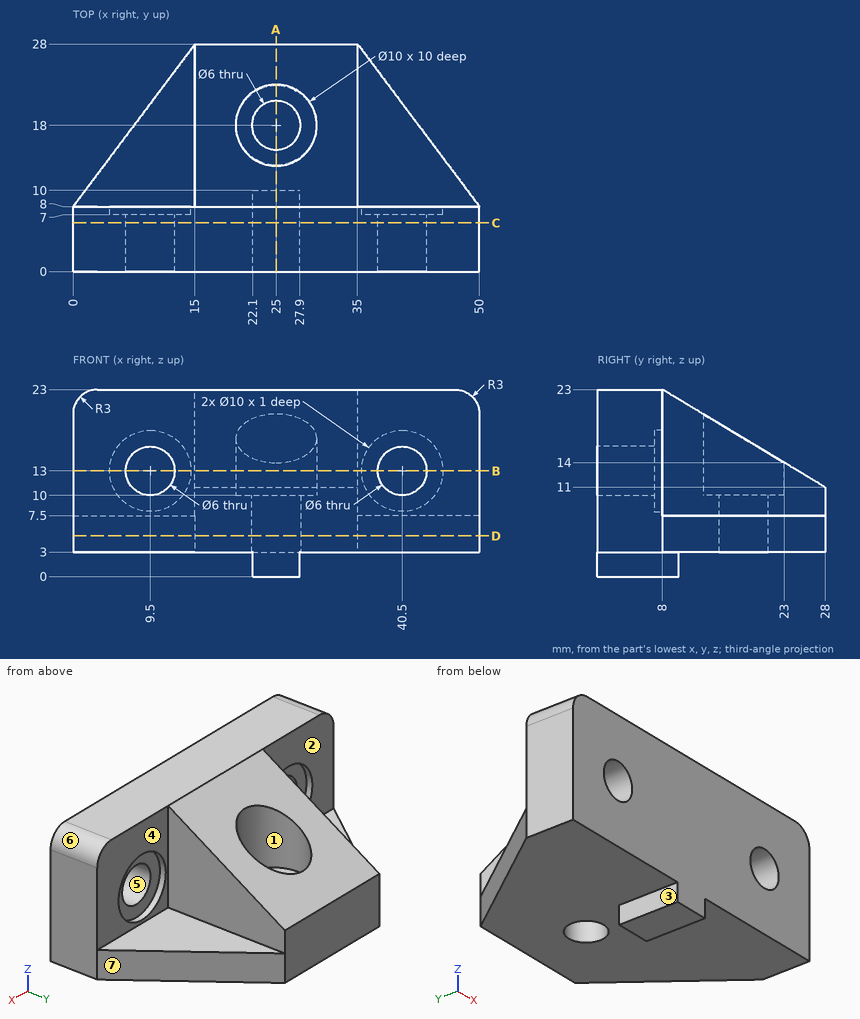
For this review, use the dimensioned drawing (mm, ordinates from the lowest corner) and the shaded views. A direction names the side the tool comes from. Give positions to 0.01 mm unless a question says otherwise; leave off trailing zeros. Order: outer loops, then holes, each group sorted by start corner. A loop starts at its lowest first (then second) coordinate and runs counter-clockwise, first axis right, second up. Notation, with made-up numbers: (38.25, -28) -> (89.25, -28) arc R18 ccw to (89.25, -2) -> close; hole circle Ø4 at (-35.75, 24). An arc over 180 degrees is marked (long way). Write item = value, one per line. Start each with the question number.
(1) For L1, parallel to X at y = 4, z = 13; L2, parallel to X at y = 14, z = 17.75; L3, parallel to Z at x = 21.5, y = 5.25, list the stretches that pass through material, from the lowest coordinate up. Write a range as from..to.
(2) For pin 1 Ø1.5 at (x, z) = (24.5, 2) entering from +Y; pin 2 Ø3 at (x, z) = (9.5, 15) entering from +Y; pin 3 Ø12 at (x, y) = (8, 20) entering from +Z; pin 4 Ø3 at (x, z) = (42.5, 10.5) entering from -Y, all flat-tipped, find the tip position at first contact; note any pin that passes through.
(3) Take a section at C-C (y = 6). Write out the cut boundary in (x, z).
(4) Tool access review of the marked faces 1, 2, 3 and 4: name each direction out of +Z, -Z, +X, -X, +Y, -Y from which nothing blocks a thin tool from reaching the whole face with its end or side.
(5) Take a section at D-D (z = 5). Write out the cut boundary in (x, y).
(6) Take a section at B-B (z = 13). Write out the cut boundary in (x, y).
(7) Take a section at A-A (x = 25). Write out the cut boundary in (y, z).
(8) Draft analysis for pull direction Z (two halves, no side actions). For the marked faces 5, 6 and 7, state which applies: +Z half, -Z half, draft (parallel to the pull), parting line (faces both ways), or undercut.
Returned:
q1.L1 = 0..6.5, 12.5..37.5, 43.5..50
q1.L2 = 15..22, 28..35
q1.L3 = 3..23
q2.pin_1 = 10
q2.pin_2 = 7
q2.pin_3 = 7.5
q2.pin_4 = 0
q3.outline = (0, 3) -> (22.1, 3) -> (22.1, 0) -> (27.9, 0) -> (27.9, 3) -> (50, 3) -> (50, 20) arc R3 ccw to (47, 23) -> (3, 23) arc R3 ccw to (0, 20) -> close; hole circle Ø6 at (9.5, 13); hole circle Ø6 at (40.5, 13)
q4.face_1 = +Z
q4.face_2 = +Z, -X, +Y
q4.face_3 = -Z, -X, +Y, -Y
q4.face_4 = +Z, +X, +Y
q5.outline = (0, 0) -> (50, 0) -> (50, 8) -> (35, 28) -> (15, 28) -> (0, 8) -> close; hole circle Ø6 at (25, 18)
q6.outline = (0, 0) -> (6.5, 0) -> (6.5, 7) -> (4.5, 7) -> (4.5, 8) -> (0, 8) -> close; (12.5, 0) -> (37.5, 0) -> (37.5, 7) -> (35.5, 7) -> (35.5, 8) -> (35, 8) -> (35, 24.67) -> (15, 24.67) -> (15, 8) -> (14.5, 8) -> (14.5, 7) -> (12.5, 7) -> close; (43.5, 0) -> (50, 0) -> (50, 8) -> (45.5, 8) -> (45.5, 7) -> (43.5, 7) -> close; hole circle Ø10 at (25, 18)
q7.outline = (0, 0) -> (10, 0) -> (10, 3) -> (15, 3) -> (15, 10) -> (13, 10) -> (13, 20) -> (8, 23) -> (0, 23) -> close; (21, 3) -> (28, 3) -> (28, 11) -> (23, 14) -> (23, 10) -> (21, 10) -> close
q8.face_5 = undercut
q8.face_6 = +Z half
q8.face_7 = draft
